Check sheet for the modelled part. Datum: model origin and axes. Units: mm. Round coordinates to 2 decimals unless told otherwise and drop trailing zeros. Order: outer loops, then holes, each group sorted by start corner. A loop starts at its lowest first (then second) coordinate and runs counter-clockwise, first axis right, second up. Notation, with made-up numbers: M -10.75,-39.75 L 27.25,-39.75 A14 ccw 27.25,-35.75 Z; hole C 52,4 d3. An arc over 180 degrees is marked long. One line per item, written item: value. Start each with the question number.
(1) Cross-section at D-D, the plane y = -7. Enter the section's corners in (x, z), and give its area (3 significant figures).
(2) Cross-section at A-A, the plane x = 0. Enter the section's corners in (y, z).
(3) Cross-section at C-C, the plane z = 2.6. Enter the section's corners in (x, y).
(4) Cross-section at B-B, the plane y = -17. Enter the section's corners in (x, z).
(5) Thickness scan on L1, parallel to Y at x = 8, z = 0.85; L2, parallel to Z at x = -1.75, y = 16; L3, parallel to X at y = -3, z = 0.65. Record the ranges inside material, lowest first.
from build123d import *

# Parameters (mm, degrees)
SKETCH_1_W          = 23
SKETCH_1_H          = 40
SKETCH_1_R          = 9.5
EXTRUDE_1_DEPTH     = 1
FILLET_1_R          = 2
SKETCH_3_R          = 1.15
CUT_EXTRUDE_1_DEPTH = 24.092206478
SKETCH_4_R          = 0.9
EXTRUDE_2_DEPTH     = 2
CHAMFER_1_SIZE      = 2
CHAMFER_1_SIZE_2    = 0.1


with BuildPart() as part:
    # 草图1 → 凸台-拉伸1 (new body)
    with BuildSketch(Plane.XY):
        Rectangle(SKETCH_1_W, SKETCH_1_H)
        with Locations((0, -4.5)):
            Circle(SKETCH_1_R, mode=Mode.SUBTRACT)
    extrude(amount=EXTRUDE_1_DEPTH)

    # 圆角1
    fillet_1_edges = [part.edges().sort_by_distance(p)[0] for p in [
        (11.5, -20, 0.5),
        (-11.5, -20, 0.5),
        (-11.5, 20, 0.5),
        (11.5, 20, 0.5),
    ]]
    fillet(fillet_1_edges, radius=FILLET_1_R)

    # 草图3 → 切除-拉伸1 (cut, through all)
    with BuildSketch(Plane.XY.offset(1)):
        with Locations((-8, 18)):
            Circle(SKETCH_3_R)
        with Locations((8, 18)):
            Circle(SKETCH_3_R)
        with Locations((-9, -17)):
            Circle(SKETCH_3_R)
        with Locations((9, -17)):
            Circle(SKETCH_3_R)
    extrude(amount=-CUT_EXTRUDE_1_DEPTH, mode=Mode.SUBTRACT)

    # 草图4 → 凸台-拉伸2 (add)
    with BuildSketch(Plane.XY.offset(1)):
        with Locations(Location((-8, -12, 0), (0, 0, 180))):
            Circle(SKETCH_4_R)
        with Locations(Location((8, -12, 0), (0, 0, 180))):
            Circle(SKETCH_4_R)
    extrude(amount=EXTRUDE_2_DEPTH)

    # 倒角1
    # the kernel refuses this chamfer: 2, 0.1 mm, written as the material it takes off along each edge
    with BuildSketch(Plane(origin=(-8, -12, 3), x_dir=(-1, 0, 0), z_dir=(0, 1, 0))) as chamfer_1_piece_1_section:
        Polygon((0.9, -CHAMFER_1_SIZE), (0.9 - CHAMFER_1_SIZE_2, 0), (0.9, 0), align=None)
    chamfer_1_piece_1 = revolve(axis=Axis((-8, -12, 3), (0, 0, 1)), mode=Mode.PRIVATE)
    chamfer_1_piece_1 = split(chamfer_1_piece_1, bisect_by=Plane(origin=(-7.141866516, -12, 1), z_dir=(0, 0, 1)), keep=Keep.TOP, mode=Mode.PRIVATE)
    add(chamfer_1_piece_1, mode=Mode.SUBTRACT)
    with BuildSketch(Plane(origin=(8, -12, 3), x_dir=(-1, 0, 0), z_dir=(0, 1, 0))) as chamfer_1_piece_2_section:
        Polygon((0.9, -CHAMFER_1_SIZE), (0.9 - CHAMFER_1_SIZE_2, 0), (0.9, 0), align=None)
    chamfer_1_piece_2 = revolve(axis=Axis((8, -12, 3), (0, 0, 1)), mode=Mode.PRIVATE)
    chamfer_1_piece_2 = split(chamfer_1_piece_2, bisect_by=Plane(origin=(8.858133484, -12, 1), z_dir=(0, 0, 1)), keep=Keep.TOP, mode=Mode.PRIVATE)
    add(chamfer_1_piece_2, mode=Mode.SUBTRACT)


solid = part.part
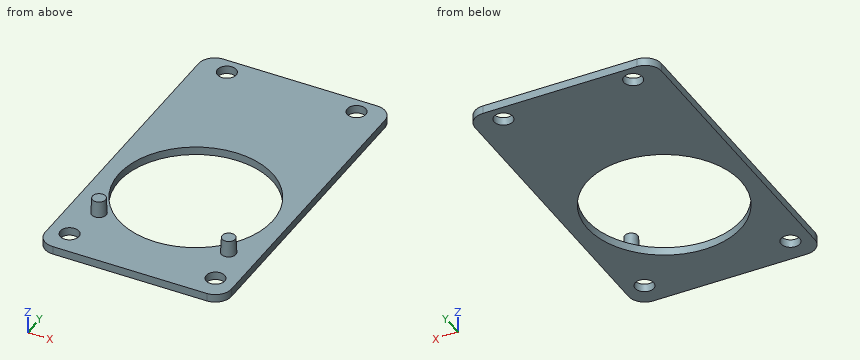
Values found:
1. outline: M -11.5,0 L -9.17,0 L -9.17,1 L -11.5,1 Z; M 9.17,0 L 11.5,0 L 11.5,1 L 9.17,1 Z
1. area: 4.67 mm^2
2. outline: M -20,0 L -14,0 L -14,1 L -20,1 Z; M 5,0 L 20,0 L 20,1 L 5,1 Z
3. outline: C -8,-12 d1.64; C 8,-12 d1.64
4. outline: M -11.5,0 L -10.15,0 L -10.15,1 L -11.5,1 Z; M -7.85,0 L 7.85,0 L 7.85,1 L -7.85,1 Z; M 10.15,0 L 11.5,0 L 11.5,1 L 10.15,1 Z
5. L1: -20 to -17.57, -16.43 to -9.62, 0.62 to 16.85, 19.15 to 20
5. L2: 0 to 1
5. L3: -11.5 to -9.38, 9.38 to 11.5
